```python
from build123d import *

# Parameters (mm, degrees)
BOSS_EXTRUDE1_DEPTH = 50
FILLET1_R           = 10
BOSS_EXTRUDE2_DEPTH = 1
BOSS_EXTRUDE3_START = 1
BOSS_EXTRUDE3_DEPTH = 1
SKETCH4_W           = 87
SKETCH4_H           = 20
CUT_EXTRUDE1_DEPTH  = 93
FILLET2_R           = 10


with BuildPart() as part:
    # Sketch1 → Boss-Extrude1 (new body)
    with BuildSketch(Plane.XY):
        Polygon((0, 0), (-77, 0), (-77, 40), (-82, 40), (-82, 0), (-102, 0), (-102, -5), (25, -5), (25, 0), (5, 0), (5, 40), (0, 40), align=None)
    extrude(amount=BOSS_EXTRUDE1_DEPTH)

    # Fillet1
    fillet1_edges = [part.edges().sort_by_distance(p)[0] for p in [
        (25, -2.5, 0),
        (25, -2.5, 50),
        (-102, -2.5, 0),
        (-102, -2.5, 50),
        (2.5, 40, 50),
        (2.5, 40, 0),
        (-79.5, 40, 0),
        (-79.5, 40, 50),
        (-82, 0, 25),
        (5, 0, 25),
    ]]
    fillet(fillet1_edges, radius=FILLET1_R - 0.0001)  # a hair under: the kernel refuses the full size

    # Sketch2 → Boss-Extrude2 (add)
    with BuildSketch(Plane(origin=(-77, 0, 0), x_dir=(0, 0, -1), z_dir=(1, 0, 0))):
        with BuildLine():
            Line((0, 0), (0, 30))
            ThreePointArc((0, 30), (-2.928932188, 37.071067812), (-10, 40))
            Line((-10, 40), (-40, 40))
            ThreePointArc((-40, 40), (-47.071067812, 37.071067812), (-50, 30))
            Line((-50, 30), (-50, 0))
            Line((-50, 0), (0, 0))
        make_face()
    extrude(amount=BOSS_EXTRUDE2_DEPTH)

    # Sketch3 → Boss-Extrude3 (add)
    with BuildSketch(Plane.ZY.offset(BOSS_EXTRUDE3_START)):
        with BuildLine():
            Line((50, 0), (50, 30))
            ThreePointArc((50, 30), (47.071067812, 37.071067812), (40, 40))
            Line((40, 40), (10, 40))
            ThreePointArc((10, 40), (2.928932188, 37.071067812), (0, 30))
            Line((0, 30), (0, 0))
            Line((0, 0), (50, 0))
        make_face()
    extrude(amount=-BOSS_EXTRUDE3_DEPTH)

    # Sketch4 → Cut-Extrude1 (cut)
    with BuildSketch(Plane.XY.offset(50)):
        with Locations((-38.5, 30)):
            Rectangle(SKETCH4_W, SKETCH4_H)
    extrude(amount=-CUT_EXTRUDE1_DEPTH, mode=Mode.SUBTRACT)

    # Fillet2
    fillet2_edges = [part.edges().sort_by_distance(p)[0] for p in [
        (2, 20, 0),
        (2, 20, 50),
        (-79, 20, 0),
        (-79, 20, 50),
    ]]
    fillet(fillet2_edges, radius=FILLET2_R)


solid = part.part
```
Geometry: final body of the model. Coordinates: model frame, mm. A direction names the side the tool comes from. Give positions to 0.01 mm unless a question says otherwise; leave off trailing zeros. Order: outer loops, then holes, each group sorted by start corner. A loop starts at its lowest first (then second) coordinate and runs counter-clockwise, first axis right, second up. Notation, with made-up numbers: M -24,30 L 19,30 A18 ccw 19,59 Z; hole C 10.5,24.5 d1. An arc over 180 degrees is marked long. Answer as CSV lines item,"result". Start each with the question number.
1) First-contact query: P1, Ø4, axis at y = 11, z = 20.5, coming from the +X side; P2, Ø1, axis at y = 2.5, z = 42.5, coming from the -X side; P3, Ø3, axis at x = -97.5, z = 28, coming from the +Y side. Flat tips, straight axial feed; report the tip coordinate or a pass-through.
2) Line query: line 1 (X direction, y = 18.25, z = 10.5); line 2 (Y direction, x = -31, z = 46.5); line 3 (X direction, y = 6.5, z = 16). Output: solid intervals per line, ascending. Write a range as from..to.
3) Cut plane C-C (x = -40). Output: boundary loops of the cut face in (y, z), then the cut area to 3 significant figures.
4) Cut plane B-B (z = 15). Output: boundary loops of the cut face in (x, y), then the cut area to 3 significant figures.
5) Set-up query: faces 4 (the flat face through (-97, 0, 25)), 5 (the flat face through (-76, 10, 25)), 6 (the flat face through (-79, 20, 25)), 7 (the flat face through (5, 15, 25)), 8 (the cylindrical face through (-78.96, 16.99, 47.15)). Return all of +Z, -Z, +X, -X, +Y, -Y with unobstructed straight access to the full face (end or side cutting, diameter ignored); none if empty.
6) Cut plane A-A (y = 13.75). Output: boundary loops of the cut face in (x, z), then the cut area to 3 significant figures.
7) Cut plane D-D (y = 4.75). Output: boundary loops of the cut face in (x, z), then the cut area to 3 significant figures.
8) Mould query, pull axis X, two halves, no side actions, for faces 1 (the flat face through (-38, 0, 25)), 2 (the cylindrical face through (-99.15, -2.54, 46.99)), 3 (the cylindrical face through (1.96, 17.15, 3.01)). Classes: +X half, -X half, draft (parallel to the pull), parting line (faces both ways), or undercut.
Findings below:
1,P1,"stops at x = 5.05"
1,P2,"stops at x = -86"
1,P3,"stops at y = 0"
2,line 1,"x = -82..-76, -1..5"
2,line 2,"y = -5..0"
2,line 3,"x = -82.63..-76, -1..5.63"
3,outline,"M -5,0 L 0,0 L 0,50 L -5,50 Z"
3,area,"250 mm²"
4,outline,"M -102,-5 L 25,-5 L 25,0 L 15,0 A10 cw 5,10 L 5,20 L -1,20 L -1,0 L -76,0 L -76,20 L -82,20 L -82,10 A10 cw -92,0 L -102,0 Z"
4,area,"918 mm²"
5,face 4,"+Z, -Z, -X, +Y"
5,face 5,"+Z, -Z, +Y"
5,face 6,"+Z, -Z, +X, -X, +Y"
5,face 7,"+Z, -Z, +X, +Y"
5,face 8,"+Z, +X, -X, +Y"
6,outline,"M -82,0.73 L -76,0.73 L -76,49.27 L -82,49.27 Z; M -1,0.73 L 5,0.73 L 5,49.27 L -1,49.27 Z"
6,area,"582 mm²"
7,outline,"M -83.49,0 L -76,0 L -76,50 L -83.49,50 Z; M -1,0 L 6.49,0 L 6.49,50 L -1,50 Z"
7,area,"749 mm²"
8,face 1,"undercut"
8,face 2,"-X half"
8,face 3,"draft"
